from build123d import *

# Parameters (mm, degrees)
IZIM1_R                     = 7.5
Y_KSEKLIK_EKSTR_ZYON1_DEPTH = 38
KES_EKSTR_ZYON1_DEPTH       = 9.5
KES_EKSTR_ZYON3_DEPTH       = 25
KES_EKSTR_ZYON4_START       = -8
IZIM4_R                     = 7.5
IZIM4_R_2                   = 6
KES_EKSTR_ZYON4_DEPTH       = 8
RADYUS1_R                   = 3
KES_EKSTR_ZYON5_DEPTH       = 10
KES_EKSTR_ZYON6_DEPTH       = 25
KES_EKSTR_ZYON7_DEPTH       = 25


with BuildPart() as part:
    # Çizim1 → Yükseklik-Ekstrüzyon1 (new body)
    with BuildSketch(Plane.XY):
        Circle(IZIM1_R)
    extrude(amount=Y_KSEKLIK_EKSTR_ZYON1_DEPTH)

    # Çizim2 → Kes-Ekstrüzyon1 (cut)
    with BuildSketch(Plane.XY.offset(38)):
        with BuildLine():
            Line((0, -1.35), (-2.734958866, -1.35))
            ThreePointArc((-2.734958866, -1.35), (0, 3.05), (2.734958866, -1.35))
            Line((2.734958866, -1.35), (0, -1.35))
        make_face()
    extrude(amount=-KES_EKSTR_ZYON1_DEPTH, mode=Mode.SUBTRACT)

    # Çizim3 → Kes-Ekstrüzyon3 (cut)
    with BuildSketch(Plane(origin=(0, 0, 0), x_dir=(-1, 0, 0), z_dir=(0, 0, -1))):
        with BuildLine():
            Line((0, -2.05), (-3.258834147, -2.05))
            ThreePointArc((-3.258834147, -2.05), (0, 3.85), (3.258834147, -2.05))
            Line((3.258834147, -2.05), (0, -2.05))
        make_face()
    extrude(amount=-KES_EKSTR_ZYON3_DEPTH, mode=Mode.SUBTRACT)

    # Çizim4 → Kes-Ekstrüzyon4 (cut)
    with BuildSketch(Plane.XY.offset(38).offset(KES_EKSTR_ZYON4_START)):
        Circle(IZIM4_R)
        Circle(IZIM4_R_2, mode=Mode.SUBTRACT)
    extrude(amount=KES_EKSTR_ZYON4_DEPTH, mode=Mode.SUBTRACT)

    # Radyus1
    # the kernel refuses this fillet: 3 mm, written as the material it adds along each edge
    with BuildSketch(Plane(origin=(0, 0, 30), x_dir=(1, 0, 0), z_dir=(0, -1, 0))) as radyus1_piece_1:
        with BuildLine():
            CenterArc((9, 2.598076211), RADYUS1_R, 180, 60)
            Line((6, 2.598076211), (5.94, 2.598076211))
            Line((5.94, 2.598076211), (5.94, 0))
            Line((5.94, 0), (6, -0.06))
            ThreePointArc((6, -0.06), (6.75, -0.06), (7.47, -0.051961524))
            Line((7.47, -0.051961524), (7.5, 0))
        make_face()
    revolve(axis=Axis((0, 0, 30), (0, 0, 1)))

    # Çizim5 → Kes-Ekstrüzyon5 (cut)
    with BuildSketch(Plane.XY.offset(38)):
        with BuildLine():
            Line((-3.120496755, -1.35), (3.120496755, -1.35))
            ThreePointArc((3.120496755, -1.35), (0, 3.4), (-3.120496755, -1.35))
        make_face()
    extrude(amount=-KES_EKSTR_ZYON5_DEPTH, mode=Mode.SUBTRACT)

    # Çizim6 → Kes-Ekstrüzyon6 (cut)
    with BuildSketch(Plane(origin=(0, 0, 0), x_dir=(-1, 0, 0), z_dir=(0, 0, -1))):
        with BuildLine():
            Line((-3.434748899, -2.05), (3.434748899, -2.05))
            ThreePointArc((3.434748899, -2.05), (0, 4), (-3.434748899, -2.05))
        make_face()
    extrude(amount=-KES_EKSTR_ZYON6_DEPTH, mode=Mode.SUBTRACT)

    # Çizim8 → Kes-Ekstrüzyon7 (cut)
    with BuildSketch(Plane(origin=(0, 0, 0), x_dir=(-1, 0, 0), z_dir=(0, 0, -1))):
        with BuildLine():
            Line((-3.893263413, -2.05), (3.893263413, -2.05))
            ThreePointArc((3.893263413, -2.05), (0, 4.4), (-3.893263413, -2.05))
        make_face()
    extrude(amount=-KES_EKSTR_ZYON7_DEPTH, mode=Mode.SUBTRACT)


solid = part.part
Read the model definition and answer for the solid it produces. Units are mm, in the model's axes. A direction names the side the tool comes from. Round coordinates to 2 decimals unless told otherwise and drop trailing zeros. Write each loop counter-clockwise with the first axis right and the second up, starting at its lowest first coordinate (ties: lowest second). Pieces come first, ordered by that corner, then holes. Notation, with made-up numbers: (-35.5, 32.25) - (20.5, 32.25) arc R26 cw to (20.5, 50.25) - close; hole circle Ø6 at (77, 40.5). An arc over 180 degrees is marked (long way). One line per question, with ' | ' between items. Start each with the question number.
1. Section D-D (z = 36) is taken. Determine the outline of the cut face in (x, y), and give its area (3 significant figures).
2. Section C-C (y = 0) is taken. Determine the outline of the cut face in (x, z), and give its area (3 significant figures).
3. Each of these flat-tipped pins is pushed along its axis until it touches: pin 1 (6 mm diameter, centred on x = 4, z = 22, fed in from -Y); pin 2 (1 mm diameter, centred on x = 1, z = 29, fed in from +Y); pin 3 (5 mm diameter, centred on x = -1, z = 34.5, fed in from +Y). Where does it stop, or does it pass through?
4. Find the intervals of material crossed by probe 1 along Y at (x, z) = (0, 12.5); probe 2 along Z at (x, y) = (-0.5, -1); probe 3 along X at (y, z) = (3.75, 8), in increasing order. Write a range as [from, to].
5. For faces 4 (the face through (0.1, 3.4, 33.1)), 5 (the face through (0, -3, 0)), 6 (the face through (0, -2.05, 12)), determine the directions among +Z, -Z, +X, -X, +Y, -Y from which every point of the face is accessible in a straight line to the end or side of a thin tool.
6. For a pull along X with two mould halves and no side action, classify faces 1 (the face through (-7.493, 0.33, 14.79)), 2 (the face through (0, -1.35, 33)), 3 (the face through (0, -3, 38)) as +X half, -X half, draft (parallel to the pull), parting line (faces both ways), or undercut.
7. Section A-A (z = 19.5) is taken. Determine the outline of the cut face in (x, y).
8. Section B-B (x = 0) is taken. Determine the outline of the cut face in (y, z), and give its area (3 significant figures).
Filled in:
1) outline: circle Ø12 at (0, 0); hole (-3.12, -1.35) - (3.12, -1.35) arc R3.4 ccw (long way) to start | area: 86.0 mm²
2) outline: (-7.5, 0) - (-4.4, 0) - (-4.4, 25) - (4.4, 25) - (4.4, 0) - (7.5, 0) - (7.5, 30) arc R3 cw to (6, 32.6) - (6, 38) - (3.4, 38) - (3.4, 28) - (-3.4, 28) - (-3.4, 38) - (-6, 38) - (-6, 32.6) arc R3 cw to (-7.5, 30) - close | area: 260 mm²
3) pin 1: y = -7.43 | pin 2: y = 7.48 | pin 3: y = 6.03
4) probe 1: [-7.5, -2.05], [4.4, 7.5] | probe 2: [25, 28] | probe 3: [-6.5, -2.3], [2.3, 6.5]
5) face 4: +Z | face 5: -Z, +X, -X, +Y, -Y | face 6: -Z
6) face 1: parting line | face 2: undercut | face 3: draft
7) outline: circle Ø15 at (0, 0); hole (-3.89, -2.05) - (3.89, -2.05) arc R4.4 ccw (long way) to start
8) outline: (-7.5, 0) - (-2.05, 0) - (-2.05, 25) - (4.4, 25) - (4.4, 0) - (7.5, 0) - (7.5, 30) arc R3 cw to (6, 32.6) - (6, 38) - (3.4, 38) - (3.4, 28) - (-1.35, 28) - (-1.35, 38) - (-6, 38) - (-6, 32.6) arc R3 cw to (-7.5, 30) - close | area: 340 mm²
